Part model, mm, in its own coordinate system. Face numbers are marked on the shaded views. A direction names the side the tool comes from. Round coordinates to 2 decimals unless told otherwise and drop trailing zeros. Loops run counter-clockwise (first coordinate to the right, second up) from the corner with the lowest first, then second, coordinate; pieces in that order, holes last. Notation, with made-up numbers: M -15,17 L 14,17 A28 cw 14,40 Z; hole C 24,37.5 d11. An arc over 180 degrees is marked long. Answer as CSV lines item,"result". Start each with the question number.
Item 1: Wall check: line 1 (Y direction, x = 1, z = 28.85); line 2 (X direction, y = -7, z = 28.9); line 3 (Y direction, x = -6.75, z = 30.45). Give the ranges that are in metal, low to high.
Item 2: Mould opens along Y. For the marked faces 1, 2, 3 and 4 say: pulls with the +Y half, pulls with the -Y half, needs draft (parallel to the pull), parting line crosses it, or undercut.
Item 3: Drop flat-ended pins along their axis: pin 1 Ø1 at (y, z) = (-10.5, 30.5) entering from -X; pin 2 Ø1 at (x, z) = (-10.5, 30) entering from +Y; pin 3 Ø0.6 at (x, z) = (11, 30) entering from -Y. Give the stop position or say it passes through.
Item 4: Which spindle directions (+Z, -Z, +X, -X, +Y, -Y) get a long thin tool onto all of the face, cutting with end or side? Do the marked faces 5, 6, 7, 8 and 9. Say none if no direction does.
Item 5: Band-saw the part on D-D (x = 3.5). Give the cut face in (y, z).
Item 6: Band-saw the part on A-A (x = 0). Give the cut face in (y, z).
```python
from build123d import *

# Parameters (mm, degrees)
SKETCH001_R        = 12
PAD001_DEPTH       = 3
SKETCH002_W        = 2.57
SKETCH002_H        = 3.2
POCKET_DEPTH       = 5
POLARPATTERN_COUNT = 8
SKETCH003_R        = 2
POCKET001_DEPTH    = 6
FILLET_R           = 1
FILLET002_R        = 1


with BuildPart() as part:
    # Sketch001 → Pad001 (new body)
    with BuildSketch(Plane.XY.offset(28.5)):
        Circle(SKETCH001_R)
    extrude(amount=PAD001_DEPTH)

    # Sketch002 (on Face3 of Pad001) → Pocket (cut)
    with BuildSketch(Plane.XY.offset(31.5)):
        with Locations((11.125, 0)):
            Rectangle(SKETCH002_W, SKETCH002_H)
    pocket = extrude(amount=-POCKET_DEPTH, mode=Mode.SUBTRACT)

    # PolarPattern: Pocket ×8 about axis
    polarpattern_axis = Axis((0, 0, 31.5), (0, 0, 1))
    for i in range(1, POLARPATTERN_COUNT):
        add(pocket.rotate(polarpattern_axis, i * 360 / POLARPATTERN_COUNT), mode=Mode.SUBTRACT)

    # Sketch003 (on Face4 of PolarPattern) → Pocket001 (cut)
    with BuildSketch(Plane.XY.offset(31.5)):
        Circle(SKETCH003_R)
    extrude(amount=-POCKET001_DEPTH, mode=Mode.SUBTRACT)

    # Fillet
    fillet_edges = [part.edges().sort_by_distance(p)[0] for p in [
        (-2, 0, 28.5),
    ]]
    fillet(fillet_edges, radius=FILLET_R)

    # Fillet002
    fillet002_edges = [part.edges().sort_by_distance(p)[0] for p in [
        (-2, 0, 31.5),
    ]]
    fillet(fillet002_edges, radius=FILLET002_R)


solid = part.part
```
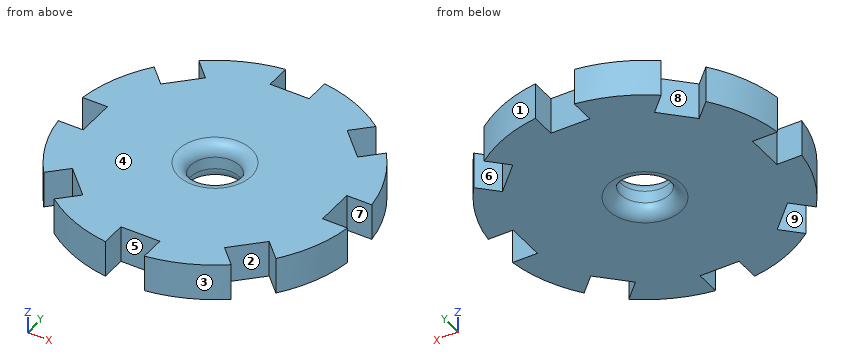
Answer block:
1,line 1,"y = -9.84 to -2, 2 to 9.84"
1,line 2,"x = -9.75 to -9.26, -6.92 to 6.92, 9.26 to 9.75"
1,line 3,"y = -9.92 to -9.01, -7.17 to 7.17, 9.01 to 9.92"
2,face 1,"pulls with the +Y half"
2,face 2,"undercut"
2,face 3,"pulls with the -Y half"
2,face 4,"needs draft"
3,pin 1,"stops at x = -6.63"
3,pin 2,"stops at y = 6.63"
3,pin 3,"stops at y = -5.43"
4,face 5,"+Z, -Z, -Y"
4,face 6,"+Z, -Z, +Y"
4,face 7,"+Z, -Z, +X"
4,face 8,"+Z, -Z"
4,face 9,"+Z, -Z, -X"
5,outline,"M -11.48,28.5 L 11.48,28.5 L 11.48,31.5 L -11.48,31.5 Z"
6,outline,"M -9.84,28.5 L -3,28.5 A1 ccw -2,29.5 L -2,30.5 A1 ccw -3,31.5 L -9.84,31.5 Z; M 2,29.5 A1 ccw 3,28.5 L 9.84,28.5 L 9.84,31.5 L 3,31.5 A1 ccw 2,30.5 Z"
